Source: CAD feature listing. Evaluate the final solid. Frame: model axes, mm. A direction names the side the tool comes from. Give positions to 0.01 mm unless a question says otherwise; leave off trailing zeros. Order: outer loops, then holes, each group sorted by start corner. A loop starts at its lowest first (then second) coordinate and runs counter-clockwise, first axis right, second up. Notation, with made-up numbers: M 54,15.25 L 62,15.25 A9 ccw 62,31.25 Z; hole C 38,-7 d4. An arc over 180 degrees is marked long. Return JSON: item names as keys, results as strings.
from build123d import *

# Parameters (mm, degrees)
SKETCH_1_W          = 181
SKETCH_1_H          = 45
EXTRUDE_1_DEPTH     = 1.5
SKETCH_2_W          = 18
SKETCH_2_H          = 15
SKETCH_2_W_2        = 20
SKETCH_2_H_2        = 30
CUT_EXTRUDE_2_DEPTH = 94.267089587
FILLET_1_R          = 5
FILLET_2_R          = 5
FILLET_3_R          = 3
SKETCH_3_W          = 1.5
SKETCH_3_H          = 45
EXTRUDE_2_DEPTH     = 5


with BuildPart() as part:
    # 草图1 → 凸台-拉伸1 (new body)
    with BuildSketch(Plane.XY):
        Rectangle(SKETCH_1_W, SKETCH_1_H)
    extrude(amount=EXTRUDE_1_DEPTH)

    # 草图2 → 切除-拉伸2 (cut, through all)
    with BuildSketch(Plane(origin=(0, 0, 0), x_dir=(-1, 0, 0), z_dir=(0, 0, -1))):
        with Locations((0, -18.592127564)):
            Rectangle(SKETCH_2_W, SKETCH_2_H)
        with Locations((48.5, -4.5)):
            Rectangle(SKETCH_2_W_2, SKETCH_2_H_2)
        with Locations((-48.5, -4.5)):
            Rectangle(SKETCH_2_W_2, SKETCH_2_H_2)
    extrude(amount=-CUT_EXTRUDE_2_DEPTH, mode=Mode.SUBTRACT)

    # 圆角1
    fillet_1_edges = [part.edges().sort_by_distance(p)[0] for p in [
        (-9, -22.5, 0.75),
        (9, -22.5, 0.75),
    ]]
    fillet(fillet_1_edges, radius=FILLET_1_R)

    # 圆角2
    fillet_2_edges = [part.edges().sort_by_distance(p)[0] for p in [
        (-9, -11.092127564, 0.75),
        (9, -11.092127564, 0.75),
    ]]
    fillet(fillet_2_edges, radius=FILLET_2_R)

    # 圆角3
    fillet_3_edges = [part.edges().sort_by_distance(p)[0] for p in [
        (38.5, -19.5, 0.75),
        (58.5, -19.5, 0.75),
        (58.5, 10.5, 0.75),
        (38.5, 10.5, 0.75),
        (-38.5, -19.5, 0.75),
        (-38.5, 10.5, 0.75),
        (-58.5, 10.5, 0.75),
        (-58.5, -19.5, 0.75),
    ]]
    fillet(fillet_3_edges, radius=FILLET_3_R)

    # 草图3 → 凸台-拉伸2 (add)
    with BuildSketch(Plane(origin=(0, 0, 0), x_dir=(-1, 0, 0), z_dir=(0, 0, -1))):
        with Locations((79.75, 0)):
            Rectangle(SKETCH_3_W, SKETCH_3_H)
        with Locations((-79.75, 0)):
            Rectangle(SKETCH_3_W, SKETCH_3_H)
    extrude(amount=-EXTRUDE_2_DEPTH)


solid = part.part
1. Section query A-A (y = 3). Return loops of the section in (x, z), then the cut area to 3 significant figures.
Evaluation:
{"outline": "M -90.5,0 L -58.5,0 L -58.5,1.5 L -79,1.5 L -79,5 L -80.5,5 L -80.5,1.5 L -90.5,1.5 Z; M -38.5,0 L 38.5,0 L 38.5,1.5 L -38.5,1.5 Z; M 58.5,0 L 90.5,0 L 90.5,1.5 L 80.5,1.5 L 80.5,5 L 79,5 L 79,1.5 L 58.5,1.5 Z", "area": "222 mm^2"}
2. Ray query, probe 1 along X at (y, z) = (-8.5, 0.9); probe 2 along X at (y, z) = (11, 1.7); probe 3 along Y at (x, z) = (-53.5, 0.6). Return the intervals inside material, ascending.
Evaluation:
{"probe 1": "x = -90.5 to -58.5, -38.5 to 38.5, 58.5 to 90.5", "probe 2": "x = -80.5 to -79, 79 to 80.5", "probe 3": "y = -22.5 to -19.5, 10.5 to 22.5"}
3. Section query C-C (x = -48.5). Return loops of the section in (y, z), then the cut area to 3 significant figures.
Evaluation:
{"outline": "M -22.5,0 L -19.5,0 L -19.5,1.5 L -22.5,1.5 Z; M 10.5,0 L 22.5,0 L 22.5,1.5 L 10.5,1.5 Z", "area": "22.5 mm^2"}
4. First-contact query: pin 1 (2 mm diameter, centred on x = -52.5, y = 13, fed in from -Z); pin 2 (8 mm diameter, centred on x = -85, y = 3.5, fed in from +Z); pin 3 (1.8 mm diameter, centred on y = -11, z = 3, fed in from +X); pin 4 (0.8 mm diameter, centred on x = -1.5, z = 0.5, fed in from -Y). Flat tips, straight axial feed; report the tip coordinate or a pass-through.
Evaluation:
{"pin 1": "stops at z = 0", "pin 2": "stops at z = 1.5", "pin 3": "stops at x = 80.5", "pin 4": "stops at y = -11.09"}
5. Set-up query: faces 4 (the face through (-57.6, 9.64, 0.76)), 5 (the face through (-52, -22.5, 1)), 6 (the face through (-79, 0, 3)), 7 (the face through (-10.5, -21.07, 0.76)), 8 (the face through (85, 0, 1.5)). Return all of +Z, -Z, +X, -X, +Y, -Y with unobstructed straight access to the full face (end or side cutting, diameter ignored); none if empty.
Evaluation:
{"face 4": "+Z, -Z", "face 5": "+Z, -Z, +X, -X, -Y", "face 6": "+Z, +Y, -Y", "face 7": "+Z, -Z, -Y", "face 8": "+Z, +X, +Y, -Y"}
6. Section query D-D (y = -13.5). Return loops of the section in (x, z), then the cut area to 3 significant figures.
Evaluation:
{"outline": "M -90.5,0 L -58.5,0 L -58.5,1.5 L -79,1.5 L -79,5 L -80.5,5 L -80.5,1.5 L -90.5,1.5 Z; M -38.5,0 L -8.28,0 L -8.28,1.5 L -38.5,1.5 Z; M 8.28,0 L 38.5,0 L 38.5,1.5 L 8.28,1.5 Z; M 58.5,0 L 90.5,0 L 90.5,1.5 L 80.5,1.5 L 80.5,5 L 79,5 L 79,1.5 L 58.5,1.5 Z", "area": "197 mm^2"}
7. Section query B-B (z = 3.7). Return loops of the section in (x, y).
Evaluation:
{"outline": "M -80.5,-22.5 L -79,-22.5 L -79,22.5 L -80.5,22.5 Z; M 79,-22.5 L 80.5,-22.5 L 80.5,22.5 L 79,22.5 Z"}
8. Draft query along X for faces 1 (the face through (57.64, 9.6, 0.76)), 2 (the face through (19, 22.5, 1)), 3 (the face through (-80.5, 0, 3)). Return one class per face: pulls with the +X half, pulls with the -X half, needs draft (parallel to the pull), parting line crosses it, or undercut.
Evaluation:
{"face 1": "undercut", "face 2": "needs draft", "face 3": "pulls with the -X half"}
